Read the model definition and answer for the solid it produces. Units are mm, in the model's axes. A direction names the side the tool comes from. Round coordinates to 2 decimals unless told otherwise and drop trailing zeros. Loops run counter-clockwise (first coordinate to the right, second up) from the corner with the lowest first, then second, coordinate; pieces in that order, holes last. Notation, with made-up numbers: (83, 46.25) - (93, 46.25) arc R21 ccw to (93, 56.25) - close; hole circle Ø11 at (36.25, -23.75). An arc over 180 degrees is marked (long way). Use CSV: the item, a comma, the result in double quotes. Start each with the question number.
1. Consider line 1 along Z through (x, y) = (-11.5, 0) (3 decimals); line 2 along X through (y, z) = (4, 23.5); line 3 along X through (y, z) = (-3.5, 22.5). Determine where each line is inside the solid, lowest interval first.
2. Find section A-A (x = -11). Give the vertices of the cut face in (y, z) (3 decimals), and give its area (3 significant figures).
3. Find section C-C (y = -1.5). Give the vertices of the cut face in (x, z) (3 decimals), and give its area (3 significant figures).
4. Find section D-D (x = 6.75). Give the vertices of the cut face in (y, z) (3 decimals), and give its area (3 significant figures).
5. A tool of negligible diameter and unlimited length cuts with its end or side. For faces 3 (the flat face through (11.135, 7.326, 13.153)), 4 (the flat face through (2, -11, 14.288)), 5 (the flat face through (0.33, 6.94, 1.57)), from which of +Z, -Z, +X, -X, +Y, -Y can it reach the whole face along a straight path? Write none if from no direction.
6. Find section B-B (z = 2.75). Give the vertices of the cut face in (x, y) (3 decimals), and give its area (3 significant figures).
7. Determine the mould class of faces 1 (the flat face through (-7, 11, 4.101)), 2 (the cylindrical face through (-11.135, 5.543, 8.45)) for opening direction Y: +Y half, -Y half, draft (parallel to the pull), parting line (faces both ways), or undercut.
from build123d import *

# Parameters (mm, degrees)
F0_W      = 25.4
F0_H      = 25.4
F1_DEPTH  = 25.4
F2_R      = 9.525
F2_R_2    = 6.985
F3_DEPTH  = 3.175
F5_DEPTH  = 3.175
F7_DEPTH  = 3.175
F9_DEPTH  = 3.175
F11_DEPTH = 3.175
F13_DEPTH = 3.175


with BuildPart() as f1:
    # F0 (on Top) → F1 (new body)
    with BuildSketch(Plane.XY):
        Rectangle(F0_W, F0_H)
    extrude(amount=F1_DEPTH)

    # F2 (on face) → F3 (cut)
    with BuildSketch(Plane(origin=(-12.7, 0, 0), x_dir=(0, -1, 0), z_dir=(-1, 0, 0))):
        with Locations((0, 12.7)):
            Circle(F2_R)
        with Locations((0, 12.7)):
            Circle(F2_R_2, mode=Mode.SUBTRACT)
    extrude(amount=-F3_DEPTH, mode=Mode.SUBTRACT)

    # F4 (on face) → F5 (cut)
    with BuildSketch(Plane(origin=(0, 12.7, 0), x_dir=(-1, 0, 0), z_dir=(0, 1, 0))):
        Polygon((8.506033, 4.101141), (0, 22.612056), (-8.506033, 4.101141), (-5.504938, 4.101141), (-3.2258, 9.061024), (0, 9.061024), (3.2258, 9.061024), (5.504938, 4.101141), align=None)
        Polygon((-2.050918, 11.50054), (0, 15.963769), (2.050918, 11.50054), (0, 11.50054), align=None, mode=Mode.SUBTRACT)
    extrude(amount=-F5_DEPTH, mode=Mode.SUBTRACT)

    # F6 (on face) → F7 (cut)
    with BuildSketch(Plane.YZ.offset(12.7)):
        Polygon((-7.62, 19.591412), (-8.928736, 19.591412), (-5.768185, 6.891412), (0, 17.024274), (5.768185, 6.891412), (8.928736, 19.591412), (7.62, 19.591412), (5.30208, 10.277347), (0, 19.591412), (-5.30208, 10.277347), align=None)
    extrude(amount=-F7_DEPTH, mode=Mode.SUBTRACT)

    # F8 (on face) → F9 (cut)
    with BuildSketch(Plane.XZ.offset(12.7)):
        Polygon((6.35, 23.8125), (-6.35, 23.8125), (-6.35, 1.5875), (6.35, 1.5875), (6.35, 4.7625), (-3.175, 4.7625), (-3.175, 11.1125), (6.35, 11.1125), (6.35, 14.2875), (-3.175, 14.2875), (-3.175, 20.6375), (6.35, 20.6375), align=None)
    extrude(amount=-F9_DEPTH, mode=Mode.SUBTRACT)

    # F10 (on face) → F11 (cut)
    with BuildSketch(Plane.XY.offset(25.4)):
        with BuildLine():
            Line((-4.504769, 9.525), (-7.679769, 9.525))
            Line((-7.679769, 9.525), (-7.679769, 0))
            ThreePointArc((-7.679769, 0), (-5.430417, -5.430417), (0, -7.679769))
            ThreePointArc((0, -7.679769), (5.430417, -5.430417), (7.679769, 0))
            Line((7.679769, 0), (7.679769, 9.525))
            Line((7.679769, 9.525), (4.504769, 9.525))
            Line((4.504769, 9.525), (4.504769, 0))
            ThreePointArc((4.504769, 0), (3.185353, -3.185353), (0, -4.504769))
            ThreePointArc((0, -4.504769), (-3.185353, -3.185353), (-4.504769, 0))
            Line((-4.504769, 0), (-4.504769, 9.525))
        make_face()
    extrude(amount=-F11_DEPTH, mode=Mode.SUBTRACT)

    # F12 (on face) → F13 (cut)
    with BuildSketch(Plane(origin=(0, 0, 0), x_dir=(1, 0, 0), z_dir=(0, 0, -1))):
        Polygon((-5.088263, 7.62), (-7.530533, 7.62), (-7.530533, -10.16), (-5.088263, -10.16), (-5.088263, -3.81), (5.910259, -10.16), (5.910259, -6.985), (-5.088263, -0.635), (5.910259, 5.715), (5.910259, 8.89), (-5.088263, 2.54), align=None)
    extrude(amount=-F13_DEPTH, mode=Mode.SUBTRACT)


solid = f1.part
Filled sheet:
1,line 1,"z = 0 to 3.175, 5.715 to 19.685, 22.225 to 25.4"
1,line 2,"x = -12.7 to -7.68, -4.5 to 4.5, 7.68 to 12.7"
1,line 3,"x = -12.7 to -6.84, -2.84 to 2.84, 6.84 to 12.7"
2,outline,"(-12.7, 0) - (12.7, 0) - (12.7, 25.4) - (-12.7, 25.4) - close; circle Ø13.97 at (0, 12.7); hole circle Ø19.05 at (0, 12.7)"
2,area,"513 mm²"
3,outline,"(-12.7, 0) - (-7.531, 0) - (-7.531, 3.175) - (-1.39, 3.175) - (-1.39, 0) - (12.7, 0) - (12.7, 14.389) - (9.525, 14.389) - (9.525, 16.956) - (12.7, 16.956) - (12.7, 25.4) - (7.532, 25.4) - (7.532, 22.225) - (4.248, 22.225) - (4.248, 25.4) - (-4.248, 25.4) - (-4.248, 22.225) - (-7.532, 22.225) - (-7.532, 25.4) - (-12.7, 25.4) - (-12.7, 22.106) - (-9.525, 22.106) - (-9.525, 19.522) - (-12.7, 19.522) - (-12.7, 5.878) - (-9.525, 5.878) - (-9.525, 3.294) - (-12.7, 3.294) - close"
3,area,"580 mm²"
4,outline,"(-12.7, 0) - (12.7, 0) - (12.7, 4.101) - (9.525, 4.101) - (9.525, 7.923) - (12.7, 7.923) - (12.7, 25.4) - (9.525, 25.4) - (9.525, 22.225) - (-3.663, 22.225) - (-3.663, 25.4) - (-12.7, 25.4) - close"
4,area,"591 mm²"
5,face 3,"+X"
5,face 4,"-Y"
5,face 5,"-Z"
6,outline,"(-12.7, -12.7) - (-6.35, -12.7) - (-6.35, -9.525) - (6.35, -9.525) - (6.35, -12.7) - (12.7, -12.7) - (12.7, 12.7) - (-12.7, 12.7) - close; hole (-7.531, -7.62) - (-5.088, -7.62) - (-5.088, -2.54) - (5.91, -8.89) - (5.91, -5.715) - (-5.088, 0.635) - (5.91, 6.985) - (5.91, 10.16) - (-5.088, 3.81) - (-5.088, 10.16) - (-7.531, 10.16) - close"
6,area,"492 mm²"
7,face 1,"draft"
7,face 2,"undercut"
